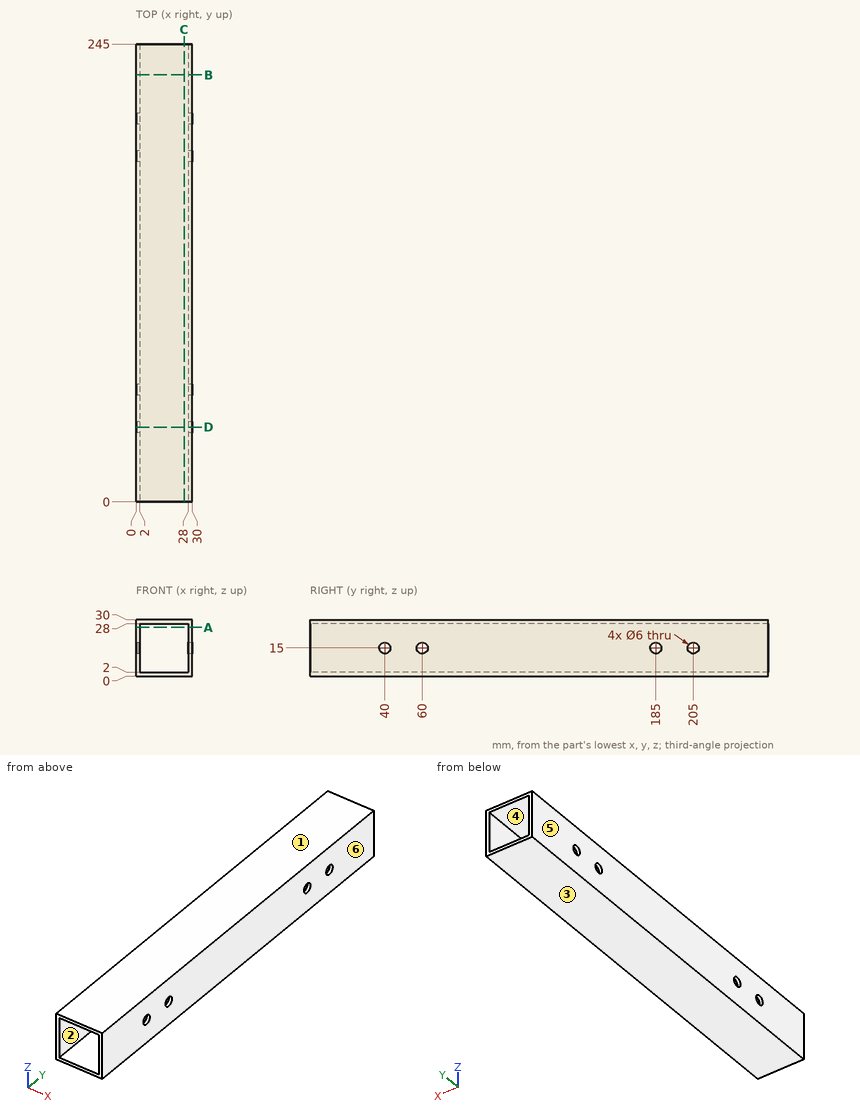
Part print with two shaded views. Sizes in mm from the minimum x, y, z corner. A direction names the side the tool comes from. Coordinates: 2 decimals unless noted, no trailing zeros. Write each loop counter-clockwise with the first axis right and the second up, starting at its lowest first coordinate (ties: lowest second). Pieces come first, ordered by that corner, then holes. Notation, with made-up numbers: (7.25, -30.5) - (59.25, -30.5) arc R12 ccw to (59.25, -23.5) - close; hole circle Ø9 at (0, 39). An arc over 180 degrees is marked (long way). One line per item, written item: value. Start each with the question number.
1. Tool access for the marked faces 1 and 2: list every direction of +Z, -Z, +X, -X, +Y, -Y with a clear straight run to the whole face (end or side of a thin tool).
2. Mould opens along X. For the marked faces 3, 4, 5 and 6 say: released by +X, released by -X, zero draft, split by the parting line, or undercut.
3. Slice it at A-A (z = 26). Write the cut outline in (x, y), plus the area to 3 significant figures.
4. Slice it at D-D (y = 40). Write the cut outline in (x, z), plus the area to 3 significant figures.
5. Slice it at B-B (y = 228.5). Write the cut outline in (x, z).
6. Probe line 1 (Y direction, x = 1.35, z = 15); line 2 (Z direction, x = 19.25, y = 211.5); line 3 (Z direction, x = 0.5, y = 185). List the from-to ranges inside material, lowest first. Write a range as from..to.
7. Slice it at C-C (x = 25.75). Write the cut outline in (y, z), plus the area to 3 significant figures.
Answers below:
1. face 1: +Z, +X, -X, +Y, -Y
1. face 2: +Y, -Y
2. face 3: zero draft
2. face 4: undercut
2. face 5: released by -X
2. face 6: released by +X
3. outline: (0, 0) - (2, 0) - (2, 245) - (0, 245) - close; (28, 0) - (30, 0) - (30, 245) - (28, 245) - close
3. area: 980 mm^2
4. outline: (0, 0) - (30, 0) - (30, 12) - (28, 12) - (28, 2) - (2, 2) - (2, 12) - (0, 12) - close; (0, 18) - (2, 18) - (2, 28) - (28, 28) - (28, 18) - (30, 18) - (30, 30) - (0, 30) - close
4. area: 200 mm^2
5. outline: (0, 0) - (30, 0) - (30, 30) - (0, 30) - close; hole (2, 2) - (28, 2) - (28, 28) - (2, 28) - close
6. line 1: y = 0..37, 43..57, 63..182, 188..202, 208..245
6. line 2: z = 0..2, 28..30
6. line 3: z = 0..12, 18..30
7. outline: (0, 0) - (245, 0) - (245, 2) - (0, 2) - close; (0, 28) - (245, 28) - (245, 30) - (0, 30) - close
7. area: 980 mm^2
